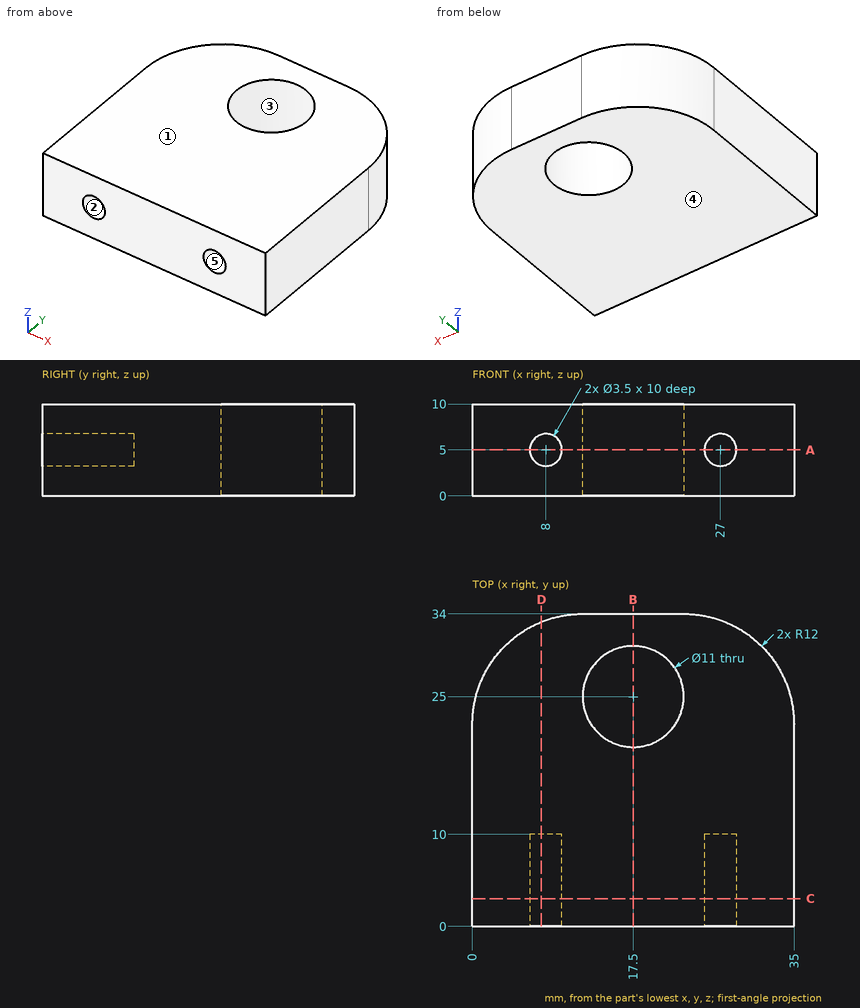
Design review of the part shown in the three views and the two pictorial views. Dimensions are in mm from the part's minimum x, y and z. A direction names the side the tool comes from. Round coordinates to 2 decimals unless told otherwise and drop trailing zeros. Loops run counter-clockwise (first coordinate to the right, second up) from the corner with the lowest first, then second, coordinate; pieces in that order, holes last. Notation, with made-up numbers: (-11, 67) - (34, 67) arc R19 ccw to (34, 82) - close; hole circle Ø9 at (-31.5, 67). An arc over 180 degrees is marked (long way). Answer as CSV lines item,"result".
(1) Consider section D-D on x = 7.5. Give the boundary of the cut face in (y, z).
Checked values:
outline,"(0, 0) - (33.12, 0) - (33.12, 10) - (0, 10) - (0, 6.68) - (10, 6.68) - (10, 3.32) - (0, 3.32) - close"
(2) Consider section C-C on y = 3. Give the boundary of the cut face in (x, z).
Checked values:
outline,"(0, 0) - (35, 0) - (35, 10) - (0, 10) - close; hole circle Ø3.5 at (8, 5); hole circle Ø3.5 at (27, 5)"
(3) Tool access review of the marked faces 1 and 2: name each direction out of +Z, -Z, +X, -X, +Y, -Y from which nothing blocks a thin tool from reaching the whole face with its end or side.
Checked values:
face 1,"+Z, +X, -X, +Y, -Y"
face 2,"-Y"
(4) Consider section A-A on z = 5. Give the boundary of the cut face in (x, y), then the cut area to 3 significant figures.
Checked values:
outline,"(0, 0) - (6.25, 0) - (6.25, 10) - (9.75, 10) - (9.75, 0) - (25.25, 0) - (25.25, 10) - (28.75, 10) - (28.75, 0) - (35, 0) - (35, 22) arc R12 ccw to (23, 34) - (12, 34) arc R12 ccw to (0, 22) - close; hole circle Ø11 at (17.5, 25)"
area,"963 mm2"
(5) Insertion check: P1, Ø4, axis at x = 8, z = 5, coming from the +Y side; P2, Ø1.8, axis at x = 27.5, z = 5, coming from the -Y side; P3, Ø2, axis at x = 4, z = 3, coming from the +Y side. Each pin has a flat end and moves straight along its axis. Give the tip position at first contact, or say it passes through.
Checked values:
P1,"stops at y = 33.83"
P2,"stops at y = 10"
P3,"stops at y = 31.75"
(6) Consider section B-B on x = 17.5. Give the boundary of the cut face in (y, z), then the cut area to 3 significant figures.
Checked values:
outline,"(0, 0) - (19.5, 0) - (19.5, 10) - (0, 10) - close; (30.5, 0) - (34, 0) - (34, 10) - (30.5, 10) - close"
area,"230 mm2"
(7) Wall thickness on line 1 (Z direction, x = 8, y = 7.5); line 2 (Y direction, x = 17.5, z = 5); line 3 (X direction, y = 2.5, z = 4.75): over which ranges is each line inside the solid? List them lowest first.
Checked values:
line 1,"z = 0 to 3.25, 6.75 to 10"
line 2,"y = 0 to 19.5, 30.5 to 34"
line 3,"x = 0 to 6.27, 9.73 to 25.27, 28.73 to 35"
(8) Mouldability with a two-part tool opening along Z and no side actions: class the marked faces 3, 4 and 5 as +Z half, -Z half, draft (parallel to the pull), parting line (faces both ways), or undercut.
Checked values:
face 3,"draft"
face 4,"-Z half"
face 5,"undercut"
